```python
from build123d import *

# Parameters (mm, degrees)
SKETCH2_W               = 163.1
SKETCH2_H               = 171.98
SKETCH2_R               = 2.5527
SKETCH2_R_2             = 1.5875
BOSS_EXTRUDE2_DEPTH     = 1.5875
FILLET1_R               = 1
CUT_EXTRUDE1_DEPTH      = 238.715061694
CUT_EXTRUDE1_DEPTH_BACK = 238.715061694
SKETCH3_R               = 3.38


with BuildPart() as part:
    # Sketch2 → Boss-Extrude2 (new body)
    with BuildSketch(Plane.XY):
        with Locations((82.55, -85.99)):
            Rectangle(SKETCH2_W, SKETCH2_H)
        with Locations((82.55, -85)):
            Circle(SKETCH2_R, mode=Mode.SUBTRACT)
        with Locations((82.55, -169.48)):
            Circle(SKETCH2_R_2, mode=Mode.SUBTRACT)
        with Locations((4.7625, -169.48)):
            Circle(SKETCH2_R_2, mode=Mode.SUBTRACT)
        with Locations((31.75, -169.48)):
            Circle(SKETCH2_R_2, mode=Mode.SUBTRACT)
        with Locations((57.15, -169.48)):
            Circle(SKETCH2_R_2, mode=Mode.SUBTRACT)
        with Locations((6.35, -94.25)):
            Circle(SKETCH2_R_2, mode=Mode.SUBTRACT)
        with Locations((6.35, -68.85)):
            Circle(SKETCH2_R_2, mode=Mode.SUBTRACT)
        with Locations((6.35, -43.45)):
            Circle(SKETCH2_R_2, mode=Mode.SUBTRACT)
        with Locations((6.35, -18.05)):
            Circle(SKETCH2_R_2, mode=Mode.SUBTRACT)
        with Locations((19.05, -3.175)):
            Circle(SKETCH2_R_2, mode=Mode.SUBTRACT)
        with Locations((44.45, -3.175)):
            Circle(SKETCH2_R_2, mode=Mode.SUBTRACT)
        with Locations((69.85, -3.175)):
            Circle(SKETCH2_R_2, mode=Mode.SUBTRACT)
        with Locations((158.75, -43.45)):
            Circle(SKETCH2_R_2, mode=Mode.SUBTRACT)
        with Locations((158.75, -18.05)):
            Circle(SKETCH2_R_2, mode=Mode.SUBTRACT)
        with Locations((146.05, -3.175)):
            Circle(SKETCH2_R_2, mode=Mode.SUBTRACT)
        with Locations((107.95, -169.48)):
            Circle(SKETCH2_R_2, mode=Mode.SUBTRACT)
        with Locations((133.35, -169.48)):
            Circle(SKETCH2_R_2, mode=Mode.SUBTRACT)
        with Locations((160.3375, -169.48)):
            Circle(SKETCH2_R_2, mode=Mode.SUBTRACT)
        with Locations((158.75, -94.25)):
            Circle(SKETCH2_R_2, mode=Mode.SUBTRACT)
        with Locations((158.75, -68.85)):
            Circle(SKETCH2_R_2, mode=Mode.SUBTRACT)
        with Locations((95.25, -3.175)):
            Circle(SKETCH2_R_2, mode=Mode.SUBTRACT)
        with Locations((120.65, -3.175)):
            Circle(SKETCH2_R_2, mode=Mode.SUBTRACT)
    extrude(amount=BOSS_EXTRUDE2_DEPTH)

    # Fillet1
    fillet1_edges = [part.edges().sort_by_distance(p)[0] for p in [
        (1, -171.98, 0.79375),
        (1, 0, 0.79375),
        (164.1, 0, 0.79375),
        (164.1, -171.98, 0.79375),
    ]]
    fillet(fillet1_edges, radius=FILLET1_R)

    # Sketch3 → Cut-Extrude1 (cut, two sides: drawn at the far end of the back side and taken through both)
    with BuildSketch(Plane.XY.offset(1.5875).offset(-CUT_EXTRUDE1_DEPTH_BACK)):
        with Locations((42.55, -146.97212)):
            Circle(SKETCH3_R)
        with Locations((82.55, -146.97212)):
            Circle(SKETCH3_R)
        with Locations((122.55, -146.97212)):
            Circle(SKETCH3_R)
    extrude(amount=CUT_EXTRUDE1_DEPTH + CUT_EXTRUDE1_DEPTH_BACK, mode=Mode.SUBTRACT)


solid = part.part
```
The listing builds one solid part. Answer for the finished solid, in the listing's coordinates (mm). Coordinates: 2 decimals unless noted, no trailing zeros. Loops run counter-clockwise (first coordinate to the right, second up) from the corner with the lowest first, then second, coordinate; pieces in that order, holes last. Notation, with made-up numbers: (60.5, 66.5) - (84.5, 66.5) arc R13 ccw to (84.5, 78.5) - close; hole circle Ø7 at (10, -39). An arc over 180 degrees is marked (long way). Use a Markdown table: item, result. Add a question column.
1) Find the intervals of material crossed by line 1 (Y direction, x = 57.5, z = 0.7); line 2 (Y direction, x = 95.25, z = 0.3), in increasing order.
2) The mould has two halves that part along X. Classify faces 1 (the cylindrical face through (44.11, -149.97, 0.78)), 2 (the flat face through (100, -85, 1.588)): released by +X, released by -X, zero draft, split by the parting line, or undercut.
3) The part is cut by section A-A, the plane y = -85. Give the vertices of the cut face in (x, z).
Here are the results:
| question | item | result |
|---|---|---|
| 1 | line 1 | y = -171.98 to -171.03, -167.93 to 0 |
| 1 | line 2 | y = -171.98 to -4.76, -1.59 to 0 |
| 2 | face 1 | undercut |
| 2 | face 2 | zero draft |
| 3 | outline | (1, 0) - (80, 0) - (80, 1.59) - (1, 1.59) - close; (85.1, 0) - (164.1, 0) - (164.1, 1.59) - (85.1, 1.59) - close |
